```python
from build123d import *

# Parameters (mm, degrees)
SKETCH_1_W      = 10
SKETCH_1_H      = 3
SKETCH_1_W_2    = 3
SKETCH_1_H_2    = 10
EXTRUDE_1_DEPTH = 3


with BuildPart() as part:
    # 草图1 → 凸台-拉伸1 (new body)
    with BuildSketch(Plane.XY):
        Polygon((-4.901841459, 22.085987353), (-4.901841459, 25.085987353), (5.098158541, 25.085987353), (5.098158541, 22.085987353), (15.098158541, 22.085987353), (15.098158541, 25.085987353), (25.098158541, 25.085987353), (25.098158541, 22.085987353), (32.598158541, 22.085987353), (32.598158541, -22.914012647), (-32.401841459, -22.914012647), (-32.401841459, 22.085987353), (-24.901841459, 22.085987353), (-24.901841459, 25.085987353), (-14.901841459, 25.085987353), (-14.901841459, 22.085987353), align=None)
        with Locations((-7.401841459, -19.414012647)):
            Rectangle(SKETCH_1_W, SKETCH_1_H, mode=Mode.SUBTRACT)
        with Locations((-22.401841459, -19.414012647)):
            Rectangle(SKETCH_1_W, SKETCH_1_H, mode=Mode.SUBTRACT)
        with Locations((7.598158541, -19.414012647)):
            Rectangle(SKETCH_1_W, SKETCH_1_H, mode=Mode.SUBTRACT)
        with Locations((22.598158541, -19.414012647)):
            Rectangle(SKETCH_1_W, SKETCH_1_H, mode=Mode.SUBTRACT)
        with Locations((-28.901841459, -7.914012647)):
            Rectangle(SKETCH_1_W_2, SKETCH_1_H_2, mode=Mode.SUBTRACT)
        with Locations((-28.901841459, 12.085987353)):
            Rectangle(SKETCH_1_W_2, SKETCH_1_H_2, mode=Mode.SUBTRACT)
        with Locations((29.098158541, -7.914012647)):
            Rectangle(SKETCH_1_W_2, SKETCH_1_H_2, mode=Mode.SUBTRACT)
        with Locations((29.098158541, 12.085987353)):
            Rectangle(SKETCH_1_W_2, SKETCH_1_H_2, mode=Mode.SUBTRACT)
    extrude(amount=EXTRUDE_1_DEPTH)


solid = part.part
```
Design review of the part built by this model. Coordinates are the model's own, in mm. A direction names the side the tool comes from. Coordinates: 2 decimals unless noted, no trailing zeros. Order: outer loops, then holes, each group sorted by start corner. A loop starts at its lowest first (then second) coordinate and runs counter-clockwise, first axis right, second up. Notation, with made-up numbers: (40, -38.75) -> (76, -38.75) arc R23 ccw to (76, -9.75) -> close; hole circle Ø11 at (14.5, 40). An arc over 180 degrees is marked (long way). One line per item, written item: value. Start each with the question number.
Q1. Tool access review of faces 4 (the flat face through (-30.402, 12, 1)), 5 (the flat face through (32.598, 0, 1)), 6 (the flat face through (5.098, 24, 1)): name each direction out of +Z, -Z, +X, -X, +Y, -Y from which nothing blocks a thin tool from reaching the whole face with its end or side.
Q2. Mouldability with a two-part tool opening along Y and no side actions: class faces 1 (the flat face through (10, 22.086, 1)), 2 (the flat face through (23, -20.914, 1)), 3 (the flat face through (-24.902, 24, 1)) as pulls with the +Y half, pulls with the -Y half, needs draft (parallel to the pull), parting line crosses it, or undercut.
Q3. Take a section at B-B, the plane x = -22. State the section outline as (y, z) points.
Q4. Take a section at C-C, the plane z = 1. Give the number of separate pieces and of enclosed holes in the cut face, then the cut area to 4 significant figures.
Q5. Take a section at A-A, the plane y = -7. State the section outline as (x, z) points, then the cut area to 3 significant figures.
Q6. For probe 1 along X at (y, z) = (11, 2.8); probe 2 along Y at (x, z) = (-27.5, 1.75); probe 3 along Y at (x, z) = (-21.5, 1.45), list the stretches that pass through material, from the lowest coordinate up.
Q7. Take a section at D-D, the plane x = -13.5. State the section outline as (y, z) points.
Q8. Insertion check: pin 1 Ø3 at (x, y) = (21, 12.5) entering from -Z. The pin has a flat end and moves straight along its axis. Give the tip position at first contact, or say it passes through.
Values follow:
1. face 4: +Z, -Z
1. face 5: +Z, -Z, +X, +Y, -Y
1. face 6: +Z, -Z, +Y
2. face 1: pulls with the +Y half
2. face 2: undercut
2. face 3: needs draft
3. outline: (-22.91, 0) -> (-20.91, 0) -> (-20.91, 3) -> (-22.91, 3) -> close; (-17.91, 0) -> (25.09, 0) -> (25.09, 3) -> (-17.91, 3) -> close
4. separate pieces: 1
4. enclosed holes: 8
4. area: 2,775 mm2
5. outline: (-32.4, 0) -> (-30.4, 0) -> (-30.4, 3) -> (-32.4, 3) -> close; (-27.4, 0) -> (27.6, 0) -> (27.6, 3) -> (-27.4, 3) -> close; (30.6, 0) -> (32.6, 0) -> (32.6, 3) -> (30.6, 3) -> close
5. area: 177 mm2
6. probe 1: x = -32.4 to -30.4, -27.4 to 27.6, 30.6 to 32.6
6. probe 2: y = -22.91 to -12.91, -2.91 to 7.09, 17.09 to 22.09
6. probe 3: y = -22.91 to -20.91, -17.91 to 25.09
7. outline: (-22.91, 0) -> (22.09, 0) -> (22.09, 3) -> (-22.91, 3) -> close
8. pin 1: stops at z = 0
